from build123d import *

# Parameters (mm, degrees)
CUT_EXTRUDE1_START = -1
SKETCH3_R          = 9.5
SKETCH3_R_2        = 8.5
CUT_EXTRUDE1_DEPTH = 1
FILLET1_R          = 1


with BuildPart() as part:
    # Sketch2 → Revolve1 (revolve)
    with BuildSketch(Plane.XY, mode=Mode.PRIVATE) as revolve1_sk:
        with BuildLine():
            Line((-6, 9.5), (-2.449489743, 9.5))
            ThreePointArc((-2.449489743, 9.5), (0, 8.5), (2.449489743, 9.5))
            Line((2.449489743, 9.5), (6, 9.5))
            Line((6, 9.5), (6, 7))
            ThreePointArc((6, 7), (5.707106781, 6.292893219), (5, 6))
            Line((5, 6), (-5, 6))
            ThreePointArc((-5, 6), (-5.707106781, 6.292893219), (-6, 7))
            Line((-6, 7), (-6, 9.5))
        make_face()
    revolve(revolve1_sk.sketch.rotate(Axis((-6, 0, 0), (1, 0, 0)), 90), axis=Axis((-6, 0, 0), (1, 0, 0)))

    # Sketch3 → Cut-Extrude1 (cut)
    with BuildSketch(Plane.ZY.offset(6).offset(CUT_EXTRUDE1_START)):
        Circle(SKETCH3_R)
        Circle(SKETCH3_R_2, mode=Mode.SUBTRACT)
    cut_extrude1 = extrude(amount=CUT_EXTRUDE1_DEPTH, mode=Mode.SUBTRACT)

    # Mirror1: Cut-Extrude1 across plane
    add(cut_extrude1.mirror(Plane(origin=(0, 0, 0), x_dir=(0, 0, 1), z_dir=(1, 0, 0))), mode=Mode.SUBTRACT)

    # Fillet1
    fillet1_edges = [part.edges().sort_by_distance(p)[0] for p in [
        (-5, 0, -8.5),
        (5, 0, -8.5),
    ]]
    fillet(fillet1_edges, radius=FILLET1_R - 0.0001)  # a hair under: the kernel refuses the full size


solid = part.part
For this review, take the finished solid that the model builds, in its own axes (mm). Coordinates: 2 decimals unless noted, no trailing zeros. Loops run counter-clockwise (first coordinate to the right, second up) from the corner with the lowest first, then second, coordinate; pieces in that order, holes last. Notation, with made-up numbers: (-11.5, -13.5) - (44.5, -13.5) arc R12 cw to (44.5, 1.5) - close; hole circle Ø5 at (58, 19.25). An arc over 180 degrees is marked (long way). Use a Markdown table: item, result. Add a question column.
Item 1: We need section C-C (x = -1.5). Give the boundary of the cut face in (y, z), and give its area (3 significant figures).
Item 2: Mouldability with a two-part tool opening along Y and no side actions: class faces 1 (the face through (6, -7, 2)), 2 (the face through (-0.07, -1.802, 5.723)), 3 (the face through (3.743, 9.274, -2.059)) as pulls with the +Y half, pulls with the -Y half, needs draft (parallel to the pull), parting line crosses it, or undercut.
Item 3: For line 1 (Z direction, x = -0.5, y = 0.75); line 2 (Z direction, x = -2, y = 2); line 3 (Y direction, x = 1.5, z = 0), list the stretches that pass through material, from the lowest coordinate up.
Item 4: Insertion check: pin 1 Ø3 at (x, z) = (-1.5, -1) entering from -Y; pin 2 Ø3 at (x, y) = (-0.5, -4) entering from -Z; pin 3 Ø1 at (y, z) = (5.5, 3) entering from -X; pin 4 Ø5.5 at (y, z) = (3.5, 1) entering from +X. Each pin has a flat end and moves straight along its axis. Give the tip position at first contact, or say it passes through.
Item 5: We need section D-D (x = 0.5). Give the boundary of the cut face in (y, z), and give its area (3 significant figures).
Results list:
| question | item | result |
|---|---|---|
| 1 | outline | circle Ø17.68 at (0, 0); hole circle Ø12 at (0, 0) |
| 1 | area | 132 mm^2 |
| 2 | face 1 | needs draft |
| 2 | face 2 | undercut |
| 2 | face 3 | parting line crosses it |
| 3 | line 1 | z = -8.5 to -5.95, 5.95 to 8.5 |
| 3 | line 2 | z = -8.91 to -5.66, 5.66 to 8.91 |
| 3 | line 3 | y = -8.84 to -6, 6 to 8.84 |
| 4 | pin 1 | stops at y = -9.5 |
| 4 | pin 2 | stops at z = -8.39 |
| 4 | pin 3 | stops at x = -5.97 |
| 4 | pin 4 | stops at x = 5.79 |
| 5 | outline | circle Ø17.07 at (0, 0); hole circle Ø12 at (0, 0) |
| 5 | area | 116 mm^2 |
